Source: CAD feature listing. Evaluate the final solid. Frame: model axes, mm. Face numbers are marked on the shaded views. A direction names the side the tool comes from. Coordinates: 2 decimals unless noted, no trailing zeros. Loops run counter-clockwise (first coordinate to the right, second up) from the corner with the lowest first, then second, coordinate; pieces in that order, holes last. Notation, with made-up numbers: (42.5, 62.5) - (86.5, 62.5) arc R9 ccw to (86.5, 74.5) - close; hole circle Ø11 at (66.5, 83). An arc over 180 degrees is marked (long way). Write item = value, one per line. Start each with the question number.
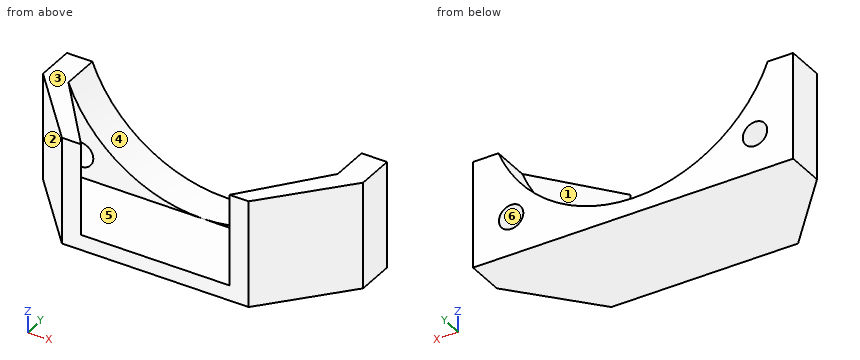
from build123d import *

# Parameters (mm, degrees)
PAD_DEPTH       = 14
SKETCH001_R     = 19
POCKET_DEPTH    = 5
POCKET001_DEPTH = 12
SKETCH003_R     = 1.6
POCKET002_DEPTH = 5
SKETCH004_W     = 42
SKETCH004_H     = 8
POCKET003_DEPTH = 14


with BuildPart() as part:
    # Sketch → Pad (new body)
    with BuildSketch(Plane(origin=(0, 0, 0), x_dir=(1, 0, 0), z_dir=(0, 0, -1))):
        Polygon((-50.823539, 3.584357), (-8.823539, 3.584357), (-8.823539, 8.584357), (-22.823539, 24.584357), (-36.823539, 24.584357), (-50.823539, 8.584357), align=None)
    extrude(amount=PAD_DEPTH)

    # Sketch001 → Pocket (cut)
    with BuildSketch(Plane(origin=(0, -3.584357, 0), x_dir=(1, 0, 0), z_dir=(0, 1, 0))):
        with Locations((-29.823539, -7)):
            Circle(SKETCH001_R)
    extrude(amount=-POCKET_DEPTH, mode=Mode.SUBTRACT)

    # Sketch002 → Pocket001 (cut)
    with BuildSketch(Plane.XY):
        Polygon((-47.487061, -8.584357), (-34.823539, -24.584357), (-24.823539, -24.584357), (-12.160017, -8.584357), align=None)
    extrude(amount=-POCKET001_DEPTH, mode=Mode.SUBTRACT)

    # Sketch003 → Pocket002 (cut)
    with BuildSketch(Plane(origin=(0, -3.584357, 0), x_dir=(1, 0, 0), z_dir=(0, 1, 0))):
        with Locations((-45.823539, 9)):
            Circle(SKETCH003_R)
        with Locations((-13.823539, 9)):
            Circle(SKETCH003_R)
    extrude(amount=-POCKET002_DEPTH, mode=Mode.SUBTRACT)

    # Sketch004 → Pocket003 (cut)
    with BuildSketch(Plane(origin=(0, 0, -14), x_dir=(1, 0, 0), z_dir=(0, 0, -1))):
        with Locations((-29.823539, 22.584357)):
            Rectangle(SKETCH004_W, SKETCH004_H)
    extrude(amount=-POCKET003_DEPTH, mode=Mode.SUBTRACT)


solid = part.part
Item 1: Cut plane D-D (y = -10). Return the cut outline in (x, z).
Item 2: Draft query along Y for the marked faces 1, 2 and 3. Return one class per face: released by +Y, released by -Y, zero draft, split by the parting line, or undercut.
Item 3: Cut plane A-A (y = -5). Return the cut outline in (x, z).
Item 4: Cut plane B-B (z = -12.5). Return the cut outline in (x, y).
Item 5: Reachability of the marked faces 4, 5 and 6 from +Z, -Z, +X, -X, +Y, -Y: full face, straight path, thin tool, end or side. Return the list, or none.
Item 6: First-contact query: pin 1 (6 mm diameter, centred on y = -12.5, z = -9, fed in from +X); pin 2 (5 mm diameter, centred on x = -23.5, y = -16, fed in from +Z). Flat tips, straight axial feed; report the tip coordinate or a pass-through.
Item 7: Material intervals for L1, parallel to X at y = -7.2, z = -9; L2, parallel to Z at x = -38.5, y = -16.75; L3, parallel to Y at x = -43, z = -11, sorted ascending. Write a range as [from, to].
Item 8: Cut plane C-C (z = -9). Return the cut outline in (x, y).
Responses:
q1.outline = (-49.58, -14) - (-10.06, -14) - (-10.06, 0) - (-13.28, 0) - (-13.28, -12) - (-46.37, -12) - (-46.37, 0) - (-49.58, 0) - close
q2.face_1 = undercut
q2.face_2 = released by -Y
q2.face_3 = zero draft
q3.outline = (-50.82, -14) - (-8.82, -14) - (-8.82, 0) - (-12.16, 0) arc R19 cw to (-47.49, 0) - (-50.82, 0) - close; hole circle Ø3.2 at (-45.82, -9); hole circle Ø3.2 at (-13.82, -9)
q4.outline = (-50.82, -8.58) - (-42.07, -18.58) - (-17.57, -18.58) - (-8.82, -8.58) - (-8.82, -3.58) - (-50.82, -3.58) - close
q5.face_4 = +Z, +Y
q5.face_5 = +Z
q5.face_6 = +Y
q6.pin_1 = -9.62
q6.pin_2 = -12
q7.L1 = [-50.82, -47.42], [-44.22, -40.07], [-19.58, -15.42], [-12.22, -8.82]
q7.L2 = [-14, -12]
q7.L3 = [-17.53, -14.25], [-8.58, -3.58]
q8.outline = (-50.82, -8.58) - (-42.07, -18.58) - (-39.57, -18.58) - (-47.49, -8.58) - (-47.42, -8.58) - (-47.42, -3.58) - (-50.82, -3.58) - close; (-44.22, -8.58) - (-40.07, -8.58) - (-40.07, -3.58) - (-44.22, -3.58) - close; (-20.07, -18.58) - (-17.57, -18.58) - (-8.82, -8.58) - (-8.82, -3.58) - (-12.22, -3.58) - (-12.22, -8.58) - (-12.16, -8.58) - close; (-19.58, -8.58) - (-15.42, -8.58) - (-15.42, -3.58) - (-19.58, -3.58) - close
